Can you work these out from the model? Positions are in its coordinate system, mm. Give positions to 0.01 mm unless a question says otherwise; leave off trailing zeros. Loops run counter-clockwise (first coordinate to the right, second up) from the corner with the lowest first, then second, coordinate; pieces in that order, holes last. Notation, with made-up numbers: (-29.5, 78) - (15.5, 78) arc R18 cw to (15.5, 104) - close; hole circle Ø3 at (22, -11.75). An arc over 180 degrees is marked (long way). Write item = value, one per line.
from build123d import *

# Parameters (mm, degrees)
CROQUIS1_W              = 40
CROQUIS1_H              = 20
CROQUIS1_R              = 2.5
SALIENTE_EXTRUIR1_DEPTH = 5
CROQUIS2_W              = 10
CROQUIS2_H              = 10
CROQUIS2_R              = 1.1
SALIENTE_EXTRUIR2_DEPTH = 5


with BuildPart() as part:
    # Croquis1 → Saliente-Extruir1 (new body)
    with BuildSketch(Plane.XY):
        Rectangle(CROQUIS1_W, CROQUIS1_H)
        with Locations((-10, 0)):
            Circle(CROQUIS1_R, mode=Mode.SUBTRACT)
        with Locations(Location((10, 0, 0), (0, 0, 180))):
            Circle(CROQUIS1_R, mode=Mode.SUBTRACT)
    extrude(amount=SALIENTE_EXTRUIR1_DEPTH)

    # Croquis2 → Saliente-Extruir2 (add)
    # profile 1 of 2: a face of its own
    with BuildSketch(Plane.XY.offset(5)):
        Polygon((5, -60), (5, -70), (20, -10), (-20, -10), (-5, -70), (-5, -60), align=None)
    # profile 2 of 2: a face of its own
    with BuildSketch(Plane.XY.offset(5)):
        with Locations((0, -65)):
            Rectangle(CROQUIS2_W, CROQUIS2_H)
        with Locations((0, -65)):
            Circle(CROQUIS2_R, mode=Mode.SUBTRACT)
    extrude(amount=-SALIENTE_EXTRUIR2_DEPTH)


solid = part.part
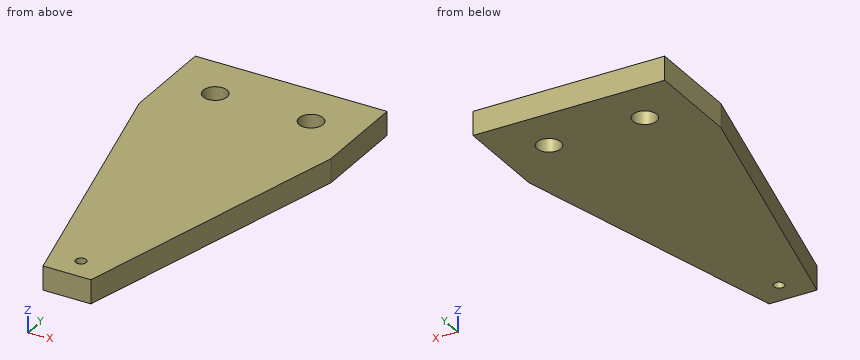
Q1. For pin 1 (1 mm diameter, centred on y = -21, z = 1, fed in from -X) (3 decimals), with a flat end and sliding along its axis, tell me the tip position at first contact or that it passes through.
Output:
pin_1 = -17.375
Q2. Imagine slicing it at B-B, the plane z = 3.45. Write out the boundary of the cut face in (x, y).
Output:
outline = (-20, -10) - (-5, -70) - (5, -70) - (20, -10) - (20, 10) - (-20, 10) - close; hole circle Ø5 at (-10, 0); hole circle Ø2.2 at (0, -65); hole circle Ø5 at (10, 0)
Q3. I need wall thicknesses on L1, parallel to Y at x = 0, z = 3.8; L2, parallel to X at y = -65.5, z = 1 (3 decimals); L3, parallel to X at y = -65, z = 2.2. Which ranges of each line are inside material? Lowest first, please.
Output:
L1 = -70 to -66.1, -63.9 to 10
L2 = -6.125 to -0.98, 0.98 to 6.125
L3 = -6.25 to -1.1, 1.1 to 6.25
Q4. Imagine slicing it at C-C, the plane y = 0. Write out the boundary of the cut face in (x, z).
Output:
outline = (-20, 0) - (-12.5, 0) - (-12.5, 5) - (-20, 5) - close; (-7.5, 0) - (7.5, 0) - (7.5, 5) - (-7.5, 5) - close; (12.5, 0) - (20, 0) - (20, 5) - (12.5, 5) - close
Q5. Imagine slicing it at D-D, the plane y = -65. Write out the boundary of the cut face in (x, z).
Output:
outline = (-6.25, 0) - (-1.1, 0) - (-1.1, 5) - (-6.25, 5) - close; (1.1, 0) - (6.25, 0) - (6.25, 5) - (1.1, 5) - close
Q6. Imagine slicing it at A-A, the plane x = 0. Write out the boundary of the cut face in (y, z).
Output:
outline = (-70, 0) - (-66.1, 0) - (-66.1, 5) - (-70, 5) - close; (-63.9, 0) - (10, 0) - (10, 5) - (-63.9, 5) - close
